The listing builds one solid part. Answer for the finished solid, in the listing's coordinates (mm). A direction names the side the tool comes from. Give positions to 0.01 mm unless a question says otherwise; leave off trailing zeros. Order: outer loops, then holes, each group sorted by start corner. A loop starts at its lowest first (then second) coordinate and runs counter-clockwise, first axis right, second up. Notation, with made-up numbers: (87.5, 47.5) - (107.5, 47.5) arc R12 ccw to (107.5, 66.5) - close; hole circle Ø8 at (4.25, 3). An arc over 180 degrees is marked (long way). Use a Markdown table: item, result. Add a question column.
1) Straight lines are drawn through the part: line 1 (X direction, y = 1.1, z = -69.5); line 2 (Z direction, x = 95, y = 0.3); line 3 (Z direction, x = -20.5, y = 1.5). For each, find the intervals that lie inside material, in ascending order.
2) Find section B-B, the plane y = 0.5. State how many separate pieces and enclosed holes the cut face has, plus the area to 3 significant figures.
3) The mould has two halves that part along Z. Classify faces 6 (the face through (-1, 0, -25)), 7 (the face through (73.72, 1.48, -73.6)), 8 (the face through (6.44, 1.52, 78.48)): released by +Z, released by -Z, zero draft, split by the parting line, or undercut.
4) For faces 1 (the face through (68.38, 1.479, 62.723)), 2 (the face through (-68.23, 1.479, 62.573)), 3 (the face through (28.923, 1.479, 70.465)), 4 (the face through (29.37, 1.48, -70.28)), 5 (the face through (73.6, 1.48, 73.72)), determine the directions among +Z, -Z, +X, -X, +Y, -Y from which every point of the face is accessible in a straight line to the end or side of a thin tool.
5) Find section A-A, the plane x = -88.5. Determine the outline of the cut face in (y, z), plus the area to 3 significant figures.
6) Find section C-C, the plane z = -37.5. Determine the outline of the cut face in (x, y).
7) Flat-ended cylindrical pins translate along their axes: pin 1 (4 mm diameter, centred on x = -70.83, z = 70.83, fed in from +Y); pin 2 (0.9 mm diameter, centred on x = -93, y = 1.5, fed in from -Z); pin 3 (1.5 mm diameter, centred on x = -27.5, y = 2.5, fed in from +Z); pin 4 (0.9 mm diameter, centred on y = 1.5, z = -96, fed in from -X). Find the tip coordinate at first contact, or state that the pin passes through.
from build123d import *

# Parameters (mm, degrees)
BOSS_EXTRUDE1_DEPTH = 3
SKETCH3_R           = 2.1
CUT_EXTRUDE1_DEPTH  = 5
FILLET1_R           = 10
SKETCH4_R           = 24
CUT_EXTRUDE2_DEPTH  = 10


with BuildPart() as part:
    # Sketch1 → Boss-Extrude1 (new body)
    with BuildSketch(Plane(origin=(0, 0, 0), x_dir=(1, 0, 0), z_dir=(0, 1, 0))):
        with BuildLine():
            ThreePointArc((36.740234303, -4), (32.740234303, 0), (36.740234303, 4))
            Line((36.740234303, 4), (76.064899264, 4))
            ThreePointArc((76.064899264, 4), (70.371903991, 29.148997043), (56.614433204, 50.957578955))
            Line((56.614433204, 50.957578955), (28.807695942, 23.150841693))
            ThreePointArc((28.807695942, 23.150841693), (23.150841693, 23.150841693), (23.150841693, 28.807695942))
            Line((23.150841693, 28.807695942), (50.957578955, 56.614433204))
            ThreePointArc((50.957578955, 56.614433204), (29.148997043, 70.371903991), (4, 76.064899264))
            Line((4, 76.064899264), (4, 36.740234303))
            ThreePointArc((4, 36.740234303), (0, 32.740234303), (-4, 36.740234303))
            Line((-4, 36.740234303), (-4, 76.064899264))
            ThreePointArc((-4, 76.064899264), (-29.148997043, 70.371903991), (-50.957578955, 56.614433204))
            Line((-50.957578955, 56.614433204), (-23.150841693, 28.807695942))
            ThreePointArc((-23.150841693, 28.807695942), (-23.150841693, 23.150841693), (-28.807695942, 23.150841693))
            Line((-28.807695942, 23.150841693), (-56.614433204, 50.957578955))
            ThreePointArc((-56.614433204, 50.957578955), (-70.371903991, 29.148997043), (-76.064899264, 4))
            Line((-76.064899264, 4), (-36.740234303, 4))
            ThreePointArc((-36.740234303, 4), (-32.740234303, 0), (-36.740234303, -4))
            Line((-36.740234303, -4), (-76.064899264, -4))
            ThreePointArc((-76.064899264, -4), (-70.371903991, -29.148997043), (-56.614433204, -50.957578955))
            Line((-56.614433204, -50.957578955), (-28.807695942, -23.150841693))
            ThreePointArc((-28.807695942, -23.150841693), (-23.150841693, -23.150841693), (-23.150841693, -28.807695942))
            Line((-23.150841693, -28.807695942), (-50.957578955, -56.614433204))
            ThreePointArc((-50.957578955, -56.614433204), (-29.148997043, -70.371903991), (-4, -76.064899264))
            Line((-4, -76.064899264), (-4, -36.740234303))
            ThreePointArc((-4, -36.740234303), (0, -32.740234303), (4, -36.740234303))
            Line((4, -36.740234303), (4, -76.064899264))
            ThreePointArc((4, -76.064899264), (29.148997043, -70.371903991), (50.957578955, -56.614433204))
            Line((50.957578955, -56.614433204), (23.150841693, -28.807695942))
            ThreePointArc((23.150841693, -28.807695942), (23.150841693, -23.150841693), (28.807695942, -23.150841693))
            Line((28.807695942, -23.150841693), (56.614433204, -50.957578955))
            ThreePointArc((56.614433204, -50.957578955), (70.371903991, -29.148997043), (76.064899264, -4))
            Line((76.064899264, -4), (36.740234303, -4))
        make_face()
        with BuildLine():
            ThreePointArc((-4, 76.064899264), (0, 76.17), (4, 76.064899264))
            Line((4, 76.064899264), (4, 100.17))
            ThreePointArc((4, 100.17), (0, 104.17), (-4, 100.17))
            Line((-4, 100.17), (-4, 76.064899264))
        make_face()
        with BuildLine():
            Line((4, 36.740234303), (4, 76.064899264))
            ThreePointArc((4, 76.064899264), (0, 76.17), (-4, 76.064899264))
            Line((-4, 76.064899264), (-4, 36.740234303))
            ThreePointArc((-4, 36.740234303), (0, 32.740234303), (4, 36.740234303))
        make_face()
        with BuildLine():
            ThreePointArc((-56.614433204, 50.957578955), (-53.860323523, 53.860323523), (-50.957578955, 56.614433204))
            Line((-50.957578955, 56.614433204), (-68.002459147, 73.659313396))
            ThreePointArc((-68.002459147, 73.659313396), (-73.659313396, 73.659313396), (-73.659313396, 68.002459147))
            Line((-73.659313396, 68.002459147), (-56.614433204, 50.957578955))
        make_face()
        with BuildLine():
            Line((-23.150841693, 28.807695942), (-50.957578955, 56.614433204))
            ThreePointArc((-50.957578955, 56.614433204), (-53.860323523, 53.860323523), (-56.614433204, 50.957578955))
            Line((-56.614433204, 50.957578955), (-28.807695942, 23.150841693))
            ThreePointArc((-28.807695942, 23.150841693), (-23.150841693, 23.150841693), (-23.150841693, 28.807695942))
        make_face()
        with BuildLine():
            ThreePointArc((-76.064899264, -4), (-76.17, 0), (-76.064899264, 4))
            Line((-76.064899264, 4), (-100.17, 4))
            ThreePointArc((-100.17, 4), (-104.17, 0), (-100.17, -4))
            Line((-100.17, -4), (-76.064899264, -4))
        make_face()
        with BuildLine():
            Line((-36.740234303, 4), (-76.064899264, 4))
            ThreePointArc((-76.064899264, 4), (-76.17, 0), (-76.064899264, -4))
            Line((-76.064899264, -4), (-36.740234303, -4))
            ThreePointArc((-36.740234303, -4), (-32.740234303, 0), (-36.740234303, 4))
        make_face()
        with BuildLine():
            Line((-68.002459147, -73.659313396), (-50.957578955, -56.614433204))
            ThreePointArc((-50.957578955, -56.614433204), (-53.860323523, -53.860323523), (-56.614433204, -50.957578955))
            Line((-56.614433204, -50.957578955), (-73.659313396, -68.002459147))
            ThreePointArc((-73.659313396, -68.002459147), (-73.659313396, -73.659313396), (-68.002459147, -73.659313396))
        make_face()
        with BuildLine():
            ThreePointArc((-56.614433204, -50.957578955), (-53.860323523, -53.860323523), (-50.957578955, -56.614433204))
            Line((-50.957578955, -56.614433204), (-23.150841693, -28.807695942))
            ThreePointArc((-23.150841693, -28.807695942), (-23.150841693, -23.150841693), (-28.807695942, -23.150841693))
            Line((-28.807695942, -23.150841693), (-56.614433204, -50.957578955))
        make_face()
        with BuildLine():
            ThreePointArc((-4, -76.064899264), (0, -76.17), (4, -76.064899264))
            Line((4, -76.064899264), (4, -36.740234303))
            ThreePointArc((4, -36.740234303), (0, -32.740234303), (-4, -36.740234303))
            Line((-4, -36.740234303), (-4, -76.064899264))
        make_face()
        with BuildLine():
            Line((4, -100.17), (4, -76.064899264))
            ThreePointArc((4, -76.064899264), (0, -76.17), (-4, -76.064899264))
            Line((-4, -76.064899264), (-4, -100.17))
            ThreePointArc((-4, -100.17), (0, -104.17), (4, -100.17))
        make_face()
        with BuildLine():
            ThreePointArc((50.957578955, -56.614433204), (53.860323523, -53.860323523), (56.614433204, -50.957578955))
            Line((56.614433204, -50.957578955), (28.807695942, -23.150841693))
            ThreePointArc((28.807695942, -23.150841693), (23.150841693, -23.150841693), (23.150841693, -28.807695942))
            Line((23.150841693, -28.807695942), (50.957578955, -56.614433204))
        make_face()
        with BuildLine():
            Line((73.659313396, -68.002459147), (56.614433204, -50.957578955))
            ThreePointArc((56.614433204, -50.957578955), (53.860323523, -53.860323523), (50.957578955, -56.614433204))
            Line((50.957578955, -56.614433204), (68.002459147, -73.659313396))
            ThreePointArc((68.002459147, -73.659313396), (73.659313396, -73.659313396), (73.659313396, -68.002459147))
        make_face()
        with BuildLine():
            Line((76.064899264, 4), (36.740234303, 4))
            ThreePointArc((36.740234303, 4), (32.740234303, 0), (36.740234303, -4))
            Line((36.740234303, -4), (76.064899264, -4))
            ThreePointArc((76.064899264, -4), (76.143720282, -2.000690266), (76.17, 0))
            ThreePointArc((76.17, 0), (76.143720282, 2.000690266), (76.064899264, 4))
        make_face()
        with BuildLine():
            Line((100.17, 4), (76.064899264, 4))
            ThreePointArc((76.064899264, 4), (76.143720282, 2.000690266), (76.17, 0))
            ThreePointArc((76.17, 0), (76.143720282, -2.000690266), (76.064899264, -4))
            Line((76.064899264, -4), (100.17, -4))
            ThreePointArc((100.17, -4), (104.17, 0), (100.17, 4))
        make_face()
        with BuildLine():
            Line((28.807695942, 23.150841693), (56.614433204, 50.957578955))
            ThreePointArc((56.614433204, 50.957578955), (53.860323523, 53.860323523), (50.957578955, 56.614433204))
            Line((50.957578955, 56.614433204), (23.150841693, 28.807695942))
            ThreePointArc((23.150841693, 28.807695942), (23.150841693, 23.150841693), (28.807695942, 23.150841693))
        make_face()
        with BuildLine():
            ThreePointArc((50.957578955, 56.614433204), (53.860323523, 53.860323523), (56.614433204, 50.957578955))
            Line((56.614433204, 50.957578955), (73.659313396, 68.002459147))
            ThreePointArc((73.659313396, 68.002459147), (73.659313396, 73.659313396), (68.002459147, 73.659313396))
            Line((68.002459147, 73.659313396), (50.957578955, 56.614433204))
        make_face()
    extrude(amount=BOSS_EXTRUDE1_DEPTH)

    # Sketch3 → Cut-Extrude1 (cut)
    with BuildSketch(Plane(origin=(0, 3, 0), x_dir=(1, 0, 0), z_dir=(0, 1, 0))):
        with Locations(Location((100.17, 0, 0), (0, 0, 270))):
            Circle(SKETCH3_R)
        with Locations(Location((70.830886271, -70.830886271, 0), (0, 0, 270))):
            Circle(SKETCH3_R)
        with Locations(Location((0, -100.17, 0), (0, 0, 270))):
            Circle(SKETCH3_R)
        with Locations(Location((-70.830886271, -70.830886271, 0), (0, 0, 270))):
            Circle(SKETCH3_R)
        with Locations(Location((-100.17, 0, 0), (0, 0, 270))):
            Circle(SKETCH3_R)
        with Locations(Location((-70.830886271, 70.830886271, 0), (0, 0, 270))):
            Circle(SKETCH3_R)
        with Locations(Location((0, 100.17, 0), (0, 0, 270))):
            Circle(SKETCH3_R)
        with Locations(Location((70.830886271, 70.830886271, 0), (0, 0, 270))):
            Circle(SKETCH3_R)
    extrude(amount=-CUT_EXTRUDE1_DEPTH, mode=Mode.SUBTRACT)

    # Fillet1
    fillet1_edges = [part.edges().sort_by_distance(p)[0] for p in [
        (76.064899264, 1.5, -4),
        (76.064899264, 1.5, 4),
        (56.614433204, 1.5, 50.957578955),
        (50.957578955, 1.5, 56.614433204),
        (4, 1.5, 76.064899264),
        (-4, 1.5, 76.064899264),
        (-50.957578955, 1.5, 56.614433204),
        (-56.614433204, 1.5, 50.957578955),
        (-76.064899264, 1.5, 4),
        (-76.064899264, 1.5, -4),
        (-56.614433204, 1.5, -50.957578955),
        (-50.957578955, 1.5, -56.614433204),
        (-4, 1.5, -76.064899264),
        (4, 1.5, -76.064899264),
        (50.957578955, 1.5, -56.614433204),
        (56.614433204, 1.5, -50.957578955),
    ]]
    fillet(fillet1_edges, radius=FILLET1_R)

    # Sketch4 → Cut-Extrude2 (cut)
    with BuildSketch(Plane(origin=(0, 3, 0), x_dir=(1, 0, 0), z_dir=(0, 1, 0))):
        Circle(SKETCH4_R)
        with BuildLine():
            Line((-25.793971814, 12.027926591), (0, 0))
            Line((0, 0), (-9.734063927, -26.744120839))
            ThreePointArc((-9.734063927, -26.744120839), (-10.54568287, -27.606769252), (-11.730108272, -27.611674341))
            ThreePointArc((-11.730108272, -27.611674341), (-27.716385975, -11.480502971), (-27.81884127, 11.229963064))
            ThreePointArc((-27.81884127, 11.229963064), (-26.977857614, 12.064009875), (-25.793971814, 12.027926591))
        make_face()
        with BuildLine():
            ThreePointArc((24, 0), (5.194550735, 23.431104171), (-21.751386889, 10.142838282))
            Line((-21.751386889, 10.142838282), (0, 0))
            Line((0, 0), (-8.20848344, -22.552622899))
            ThreePointArc((-8.20848344, -22.552622899), (13.765834472, -19.659649063), (24, 0))
        make_face()
        with BuildLine():
            Line((0, 0), (-21.751386889, 10.142838282))
            ThreePointArc((-21.751386889, 10.142838282), (-22.17310878, -9.184402377), (-8.20848344, -22.552622899))
            Line((-8.20848344, -22.552622899), (0, 0))
        make_face()
    extrude(amount=-CUT_EXTRUDE2_DEPTH, mode=Mode.SUBTRACT)


solid = part.part
The answers:
| question | item | result |
|---|---|---|
| 1 | line 1 | -74.6 to -72.46, -69.21 to -63.84, -31.17 to 31.17, 63.84 to 69.21, 72.46 to 74.6 |
| 1 | line 2 | -4 to 4 |
| 1 | line 3 | -73.36 to -12.48, 21.9 to 73.36 |
| 2 | separate pieces | 1 |
| 2 | enclosed holes | 9 |
| 2 | area | 18,000 mm2 |
| 3 | face 6 | zero draft |
| 3 | face 7 | undercut |
| 3 | face 8 | released by +Z |
| 4 | face 1 | +X, +Y, -Y |
| 4 | face 2 | -X, +Y, -Y |
| 4 | face 3 | +Z, +Y, -Y |
| 4 | face 4 | -Z, +Y, -Y |
| 4 | face 5 | +Y, -Y |
| 5 | outline | (0, -4) - (3, -4) - (3, 4) - (0, 4) - close |
| 5 | area | 24.0 mm2 |
| 6 | outline | (-66.3, 0) - (66.3, 0) - (66.3, 3) - (-66.3, 3) - close |
| 7 | pin 1 | through |
| 7 | pin 2 | z = -4 |
| 7 | pin 3 | z = 71.32 |
| 7 | pin 4 | x = -4 |
